For this review, take the finished solid that the model builds, in its own axes (mm). Face numbers are marked on the shaded views. Round coordinates to 2 decimals unless told otherwise and drop trailing zeros. Write each loop counter-clockwise with the first axis right and the second up, starting at its lowest first coordinate (ties: lowest second). Pieces come first, ordered by that corner, then holes. Notation, with made-up numbers: M -10.5,2.5 L 30.5,2.5 A17 ccw 30.5,11.5 Z; hole C 67,-39.75 d11. An arc over 180 degrees is marked long. Write each question's results on one line, items separated by ' | '. Start each with the question number.
```python
from build123d import *

# Parameters (mm, degrees)
F0_W     = 22
F0_H     = 27
F0_R     = 8.5
F1_DEPTH = 7.5
F3_DEPTH = 2
F6_DEPTH = 2


with BuildPart() as f1:
    # F0 (on Front) → F1 (new body, symmetric)
    with BuildSketch(Plane.XZ):
        Rectangle(F0_W, F0_H)
        Circle(F0_R, mode=Mode.SUBTRACT)
    extrude(amount=F1_DEPTH, both=True)

    # F2 (on face) → F3 (cut)
    with BuildSketch(Plane(origin=(0, 0, -13.5), x_dir=(1, 0, 0), z_dir=(0, 0, -1))):
        with BuildLine():
            Line((3, 7.5), (-3, 7.5))
            Line((-3, 7.5), (-3, 2.5583377574))
            ThreePointArc((-3, 2.5583377574), (0, -3.9427264781), (3, 2.5583377574))
            Line((3, 2.5583377574), (3, 7.5))
        make_face()
    extrude(amount=-F3_DEPTH, mode=Mode.SUBTRACT)

    # F5 (on offset) → F6 (cut)
    with BuildSketch(Plane(origin=(0, 0, -11.5), x_dir=(1, 0, 0), z_dir=(0, 0, -1))):
        with BuildLine():
            Line((5.5, 7.5), (-5.5, 7.5))
            Line((-5.5, 7.5), (-5.5, 2.5583377574))
            ThreePointArc((-5.5, 2.5583377574), (0, -6.0658958185), (5.5, 2.5583377574))
            Line((5.5, 2.5583377574), (5.5, 7.5))
        make_face()
    extrude(amount=-F6_DEPTH, mode=Mode.SUBTRACT)


solid = f1.part
```
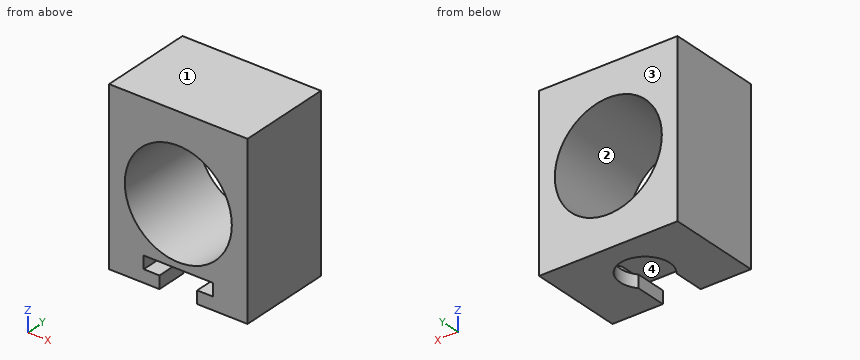
Item 1: We need section B-B on z = -5. State the section outline as (x, y) points.
Item 2: Insertion check: P1, Ø6.5, axis at x = 0, y = 0, coming from the -Z side; P2, Ø1.5, axis at x = 5, z = -10, coming from the -Y side. Each pin has a flat end and moves straight along its axis. Give the tip position at first contact, or say it passes through.
Item 3: For probe 1 along Z at (x, y) = (4, -4.75); probe 2 along Z at (x, y) = (0, 4.5); probe 3 along Z at (x, y) = (0, -3.25), list the stretches that pass through material, from the lowest coordinate up.
Item 4: We need section C-C on y = 0. State the section outline as (x, z) points.
Item 5: We need section A-A on x = 0. State the section outline as (y, z) points.
Item 6: We need section D-D on z = 0. State the section outline as (x, y) points.
Item 7: Mouldability with a two-part tool opening along Z and no side actions: class the marked faces 1, 2, 3 and 4 as pulls with the +Z half, pulls with the -Z half, needs draft (parallel to the pull), parting line crosses it, or undercut.
Numbers:
1) outline: M -11,-7.5 L -6.87,-7.5 L -6.87,7.5 L -11,7.5 Z; M 6.87,-7.5 L 11,-7.5 L 11,7.5 L 6.87,7.5 Z
2) P1: stops at z = -9.5 | P2: stops at y = -7.5
3) probe 1: z = -13.5 to -11.5, -9.5 to -7.5, 7.5 to 13.5 | probe 2: z = -13.5 to -11.5, -9.5 to -8.5, 8.5 to 13.5 | probe 3: z = -9.5 to -8.5, 8.5 to 13.5
4) outline: M -11,-13.5 L -3.94,-13.5 L -3.94,-11.5 L -6.07,-11.5 L -6.07,-9.5 L 6.07,-9.5 L 6.07,-11.5 L 3.94,-11.5 L 3.94,-13.5 L 11,-13.5 L 11,13.5 L -11,13.5 Z; hole C 0,0 d17
5) outline: M -7.5,-9.5 L 6.07,-9.5 L 6.07,-11.5 L 3.94,-11.5 L 3.94,-13.5 L 7.5,-13.5 L 7.5,-8.5 L -7.5,-8.5 Z; M -7.5,8.5 L 7.5,8.5 L 7.5,13.5 L -7.5,13.5 Z
6) outline: M -11,-7.5 L -8.5,-7.5 L -8.5,7.5 L -11,7.5 Z; M 8.5,-7.5 L 11,-7.5 L 11,7.5 L 8.5,7.5 Z
7) face 1: pulls with the +Z half | face 2: undercut | face 3: needs draft | face 4: undercut
